The model under review builds one solid part; all positions refer to its coordinate system, in mm. A direction names the side the tool comes from. Coordinates: 2 decimals unless noted, no trailing zeros. Order: outer loops, then holes, each group sorted by start corner. A loop starts at its lowest first (then second) coordinate and runs counter-clockwise, first axis right, second up. Notation, with made-up numbers: (53, 86.25) - (102, 86.25) arc R20 cw to (102, 107.25) - close; hole circle Ø1 at (61.25, 20). An arc over 180 degrees is marked (long way). Answer in a Markdown table with one row per item.
```python
from build123d import *

# Parameters (mm, degrees)
BOX012_W               = 1
BOX012_H               = 5
BOX012_DEPTH           = 6
BOX012_PLACEMENT_ANGLE = 90
BOX011_W               = 1
BOX011_H               = 5
BOX011_DEPTH           = 6
BOX011_PLACEMENT_ANGLE = 90
CYLINDER017_R          = 2.5
CYLINDER017_DEPTH      = 10


with BuildPart() as cubo008:
    # Box012 → Box012 (new body)
    with BuildSketch(Plane.XY):
        with Locations((0.5, 2.5)):
            Rectangle(BOX012_W, BOX012_H)
    extrude(amount=BOX012_DEPTH)


with BuildPart() as cubo008_1:
    # Box012 placement: moved
    add(cubo008.part.moved(Location((2.5, -2.5, 4))).rotate(Axis((2.5, -2.5, 4), (0, 0, 1)), BOX012_PLACEMENT_ANGLE))


with BuildPart() as fusion008:
    # Box011 → Box011 (new body)
    with BuildSketch(Plane.XY):
        with Locations((0.5, 2.5)):
            Rectangle(BOX011_W, BOX011_H)
    extrude(amount=BOX011_DEPTH)


with BuildPart() as fusion008_1:
    # Box011 placement: moved
    add(fusion008.part.moved(Location((2.5, 1.5, 4))).rotate(Axis((2.5, 1.5, 4), (0, 0, 1)), BOX011_PLACEMENT_ANGLE))

    # Fusion008: union Cubo008
    add(cubo008_1.part)


with BuildPart() as axis_final001:
    # Cylinder017 → Cylinder017 (new body)
    with BuildSketch(Plane.XY):
        Circle(CYLINDER017_R)
    extrude(amount=CYLINDER017_DEPTH)

    # Cut018: cut Fusion008
    add(fusion008_1.part, mode=Mode.SUBTRACT)


with BuildPart() as axis_final001_1:
    # Cut018 placement: moved
    add(axis_final001.part.moved(Location((0, 8, 19))))


solid = axis_final001_1.part
```
Item 1: To check wall thickness, follow line 1 (Z direction, x = -0.75, y = 5.8); line 2 (Y direction, x = 1.8, z = 26.5); line 3 (Y direction, x = -1.7, z = 21.25). State the ranges of each line that lie inside material, in increasing order. Write a range as from..to.
Check values:
| item | result |
|---|---|
| line 1 | 19..23 |
| line 2 | 6.5..9.5 |
| line 3 | 6.17..9.83 |
Item 2: We need section C-C, the plane y = 6.05. Write out the cut boundary in (x, z).
Check values:
| item | result |
|---|---|
| outline | (-1.56, 19) - (1.56, 19) - (1.56, 23) - (-1.56, 23) - close |
Item 3: Clearance check with flat-ended pins moving along their axes: pin 1 Ø1 at (y, z) = (6.5, 25) entering from -X; pin 2 Ø3 at (x, z) = (1, 26) entering from +Y; pin 3 Ø0.8 at (x, y) = (1, 10) entering from +Z. State where each tip first meets the part, or that it passes through.
Check values:
| item | result |
|---|---|
| pin 1 | x = -2.29 |
| pin 2 | y = 9.5 |
| pin 3 | z = 23 |
Item 4: Tool access review of faces 1 (the face through (0, 6.5, 26)), 2 (the face through (0, 10, 23)), 3 (the face through (2.385, 8.751, 22.819)): name each direction out of +Z, -Z, +X, -X, +Y, -Y from which nothing blocks a thin tool from reaching the whole face with its end or side.
Check values:
| item | result |
|---|---|
| face 1 | +Z, +X, -X, -Y |
| face 2 | +Z, +X, -X, +Y |
| face 3 | +Z, -Z |
Item 5: We need section A-A, the plane x = 0. Write out the cut boundary in (y, z).
Check values:
| item | result |
|---|---|
| outline | (5.5, 19) - (10.5, 19) - (10.5, 23) - (9.5, 23) - (9.5, 29) - (6.5, 29) - (6.5, 23) - (5.5, 23) - close |
Item 6: We need section D-D, the plane x = -1.55. Write out the cut boundary in (y, z).
Check values:
| item | result |
|---|---|
| outline | (6.04, 19) - (9.96, 19) - (9.96, 23) - (9.5, 23) - (9.5, 29) - (6.5, 29) - (6.5, 23) - (6.04, 23) - close |
Item 7: We need section B-B, the plane z = 26.25. Write out the cut boundary in (x, y).
Check values:
| item | result |
|---|---|
| outline | (-2, 6.5) - (2, 6.5) arc R2.5 ccw to (2, 9.5) - (-2, 9.5) arc R2.5 ccw to start |
